CAD build for the part. Positions are in the model's coordinates, mm. A direction names the side the tool comes from. Coordinates: 2 decimals unless noted, no trailing zeros. Order: outer loops, then holes, each group sorted by start corner. A loop starts at its lowest first (then second) coordinate and runs counter-clockwise, first axis right, second up. Notation, with made-up numbers: M -32,-11 L -8,-11 A31 ccw -8,27 Z; hole C 48,44.25 d10. An arc over 180 degrees is marked long. One line per item, written item: value.
from build123d import *

# Parameters (mm, degrees)
F1_DEPTH = 20
F0_R     = 2
F0_R_2   = 4.5
F2_DEPTH = 4
F3_R     = 2
F4_R     = 1


with BuildPart() as f1:
    # F0 (on Top) → F1 (new body)
    with BuildSketch(Plane.XY):
        Polygon((-0.5, 45), (0, 0), (31, 0), (31.1779875703, 16.0188813289), (31.5, 45), (15.5, 45), align=None)
        Polygon((28.5000000559, 15.9295856795), (2.4999999441, 15.3551234695), (2.4999999441, 29.3559876404), (28.5000000559, 29.3559876404), align=None, mode=Mode.SUBTRACT)
    extrude(amount=F1_DEPTH)

    # F0 (on Top) → F2 (join)
    with BuildSketch(Plane.XY):
        Polygon((-0.5, 45), (0, 0), (31, 0), (31.1779875703, 16.0188813289), (31.5, 45), (15.5, 45), align=None)
        Polygon((28.5000000559, 15.9295856795), (2.4999999441, 15.3551234695), (2.4999999441, 29.3559876404), (28.5000000559, 29.3559876404), align=None, mode=Mode.SUBTRACT)
        Polygon((2.4999999441, 29.3559876404), (2.4999999441, 15.3551234695), (28.5000000559, 15.9295856795), (28.5000000559, 29.3559876404), align=None)
        with Locations((7.5, 22.4111111111)):
            Circle(F0_R, mode=Mode.SUBTRACT)
        with Locations((23.5, 22.4111111111)):
            Circle(F0_R, mode=Mode.SUBTRACT)
        with Locations((15.5, 22.5)):
            Circle(F0_R_2, mode=Mode.SUBTRACT)
    extrude(amount=-F2_DEPTH)

    # F3
    f3_edges = [f1.edges().sort_by_distance(p)[0] for p in [
        (31.25, 22.5, -4),
        (15.5, 0, -4),
        (-0.25, 22.5, -4),
        (15.5, 45, -4),
    ]]
    fillet(f3_edges, radius=F3_R)

    # F4
    f4_edges = [f1.edges().sort_by_distance(p)[0] for p in [
        (15.5, 0, 20),
        (31.25, 22.5, 20),
        (-0.25, 22.5, 20),
        (15.5, 45, 20),
        (15.5, 29.355988, 20),
        (28.5, 22.642787, 20),
        (15.5, 15.642355, 20),
        (2.5, 22.355556, 20),
        (28.5, 22.642787, 0),
        (15.5, 15.642355, 0),
        (15.5, 29.355988, 0),
        (2.5, 22.355556, 0),
    ]]
    fillet(f4_edges, radius=F4_R)


solid = f1.part
Q1. Slice it at A-A (z = 15.5). List the corners of the cut face in (x, y), plus the area to 3 significant figures.
Recorded:
outline: M -0.5,45 L 0,0 L 31,0 L 31.5,45 Z; hole M 2.5,15.36 L 28.5,15.93 L 28.5,29.36 L 2.5,29.36 Z
area: 1,060 mm^2
Q2. Which spindle directions (+Z, -Z, +X, -X, +Y, -Y) get a long thin tool onto all of the face, cutting with end or side? Do faces 4 (the face through (28.215, 22.549, 0.301)), 5 (the face through (15.276, 44.699, 19.715)). Say none if no direction does.
Recorded:
face 4: +Z
face 5: +Z, +X, -X, +Y
Q3. Drill centre lines: line 1 along X through (y, z) = (18.5, 11.25); line 2 along Y through (x, z) = (11, 17.5); line 3 along Y through (x, z) = (11.5, 14). Where is each one in solid material? Low to high.
Recorded:
line 1: x = -0.21 to 2.5, 28.5 to 31.21
line 2: y = 0 to 15.54, 29.36 to 45
line 3: y = 0 to 15.55, 29.36 to 45
Q4. Pin check, flat tips, straight feed: pin 1 Ø11.5 at (x, y) = (15.5, 22.5) entering from +Z; pin 2 Ø11 at (y, z) = (25.5, 5.5) entering from +X; pin 3 Ø13 at (x, y) = (16.5, 23.5) entering from +Z; pin 4 Ø3.5 at (x, y) = (23.5, 22.41) entering from +Z. Stop position of each tip, or through.
Recorded:
pin 1: stops at z = 0
pin 2: stops at x = 31.34
pin 3: stops at z = 19.93
pin 4: passes through
Q5. Mould opens along X. For faces 1 (the face through (15.72, 0.57, -3.4)), 2 (the face through (0.04, 22.19, 19.7)), 3 (the face through (7.066, 20.459, -1.972)) say: released by +X, released by -X, zero draft, split by the parting line, or undercut.
Recorded:
face 1: zero draft
face 2: released by -X
face 3: undercut
